Part model, mm, in its own coordinate system. Coordinates: 2 decimals unless noted, no trailing zeros. Order: outer loops, then holes, each group sorted by start corner. A loop starts at its lowest first (then second) coordinate and runs counter-clockwise, first axis right, second up. Notation, with made-up numbers: M 55.5,39 L 79.5,39 A25 cw 79.5,58 Z; hole C 73,-39 d3. An arc over 180 degrees is marked long. Answer in a Markdown table with one row per item. Add a question column.
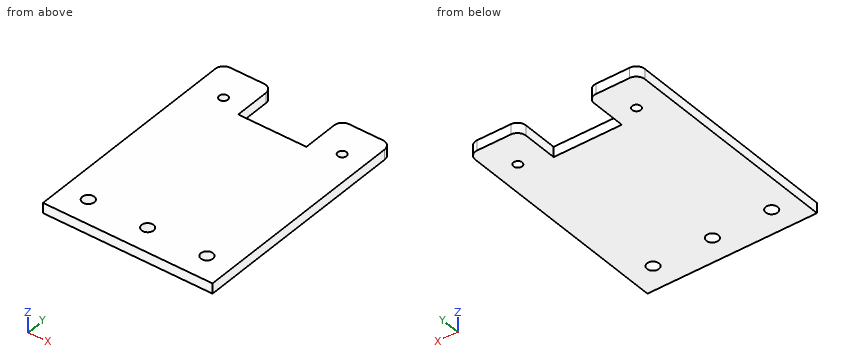
from build123d import *

# Parameters (mm, degrees)
SKETCH_1_W   = 100
SKETCH_1_H   = 135
SKETCH_1_R   = 3.525
SKETCH_1_R_2 = 2.55
PAD_DEPTH    = 6
SKETCH_W     = 40.2
SKETCH_H     = 28.5
POCKET_DEPTH = 6
FILLET_R     = 5


with BuildPart() as part:
    # Sketch_1 → Pad (new body)
    with BuildSketch(Plane.XY):
        with Locations((50, 67.5)):
            Rectangle(SKETCH_1_W, SKETCH_1_H)
        with Locations((15, 15)):
            Circle(SKETCH_1_R, mode=Mode.SUBTRACT)
        with Locations((50, 15)):
            Circle(SKETCH_1_R, mode=Mode.SUBTRACT)
        with Locations((85, 15)):
            Circle(SKETCH_1_R, mode=Mode.SUBTRACT)
        with Locations((16.629946, 115)):
            Circle(SKETCH_1_R_2, mode=Mode.SUBTRACT)
        with Locations((86.629946, 115)):
            Circle(SKETCH_1_R_2, mode=Mode.SUBTRACT)
    extrude(amount=PAD_DEPTH)

    # Sketch (on Face11 of Pad) → Pocket (cut)
    with BuildSketch(Plane.XY.offset(6)):
        with Locations((50, 123.366165)):
            Rectangle(SKETCH_W, SKETCH_H)
    extrude(amount=-POCKET_DEPTH, mode=Mode.SUBTRACT)

    # Fillet
    fillet_edges = [part.edges().sort_by_distance(p)[0] for p in [
        (0, 135, 3),
        (29.9, 135, 3),
        (70.1, 135, 3),
        (100, 135, 3),
    ]]
    fillet(fillet_edges, radius=FILLET_R)


solid = part.part
(1) Drop flat-ended pins along their axis: P1, Ø3, axis at x = 58.5, z = 2, coming from the +Y side; P2, Ø4, axis at x = 15, y = 15, coming from the +Z side. Give the stop position or say it passes through.
(2) Slice it at C-C (z = 3.85). List the corners of the cut face in (x, y) (3 decimals), and give its area (3 significant figures).
(3) Slice it at D-D (y = 15). List the corners of the cut face in (x, z) (3 decimals).
(4) Slice it at A-A (y = 115). List the corners of the cut face in (x, z), and give its area (3 significant figures).
(5) Slice it at B-B (x = 50). List the corners of the cut face in (y, z) (3 decimals), and give its area (3 significant figures).
(6) Wall check: line 1 (Y direction, x = 85, z = 1.7) (3 decimals); line 2 (X direction, y = 119, z = 4.5); line 3 (Y direction, x = 50, z = 3.3) (3 decimals). Give the ranges that are in metal, low to high.
Computed:
| question | item | result |
|---|---|---|
| 1 | P1 | stops at y = 109.12 |
| 1 | P2 | passes through |
| 2 | outline | M 0,0 L 100,0 L 100,130 A5 ccw 95,135 L 75.1,135 A5 ccw 70.1,130 L 70.1,109.116 L 29.9,109.116 L 29.9,130 A5 ccw 24.9,135 L 5,135 A5 ccw 0,130 Z; hole C 15,15 d7.05; hole C 16.63,115 d5.1; hole C 50,15 d7.05; hole C 85,15 d7.05; hole C 86.63,115 d5.1 |
| 2 | area | 12,300 mm^2 |
| 3 | outline | M 0,0 L 11.475,0 L 11.475,6 L 0,6 Z; M 18.525,0 L 46.475,0 L 46.475,6 L 18.525,6 Z; M 53.525,0 L 81.475,0 L 81.475,6 L 53.525,6 Z; M 88.525,0 L 100,0 L 100,6 L 88.525,6 Z |
| 4 | outline | M 0,0 L 14.08,0 L 14.08,6 L 0,6 Z; M 19.18,0 L 29.9,0 L 29.9,6 L 19.18,6 Z; M 70.1,0 L 84.08,0 L 84.08,6 L 70.1,6 Z; M 89.18,0 L 100,0 L 100,6 L 89.18,6 Z |
| 4 | area | 298 mm^2 |
| 5 | outline | M 0,0 L 11.475,0 L 11.475,6 L 0,6 Z; M 18.525,0 L 109.116,0 L 109.116,6 L 18.525,6 Z |
| 5 | area | 612 mm^2 |
| 6 | line 1 | y = 0 to 11.475, 18.525 to 113.039, 116.961 to 135 |
| 6 | line 2 | x = 0 to 29.9, 70.1 to 100 |
| 6 | line 3 | y = 0 to 11.475, 18.525 to 109.116 |
